```python
from build123d import *

# Parameters (mm, degrees)
MAINBLOCK_R                      = 2
MAINBLOCKBOSS_EXTRUDE1_DEPTH     = 23.4
TOPHOLECUT_SKETCH2_R             = 2.5
TOPHOLECUT_EXTRUDE1_DEPTH        = 45
MOUNTHOLEBORECUT_EXTRUDE2_DEPTH  = 2
TOPSPACERSKETCH4_R               = 3.5
TOPSPACERSKETCH4_R_2             = 2.5
TOPSPACERBOSS_EXTRUDE2_DEPTH     = 1
LOWERSPACERBOSS_EXTRUDE3_START   = 1
LOWERSPACERSKETCH5_R             = 3.5
LOWERSPACERSKETCH5_R_2           = 2.5
LOWERSPACERBOSS_EXTRUDE3_DEPTH   = 1
PUSHPINHOLESKETCH1_R             = 1
PUSHPINHOLECUT_EXTRUDE1_DEPTH    = 76.354665582
SCREWCOLLISIONSKETCH2_W          = 18.72
SCREWCOLLISIONSKETCH2_H          = 60
SCREWCOLLISIONCUT_EXTRUDE2_DEPTH = 5
SCREWCOLLISIONFILLET1_R          = 10
SCREWCOLLISIONFILLET2_R          = 10
MIDRAILINDENTSKETCH1_W           = 3.175
MIDRAILINDENTSKETCH1_H           = 40.4
MIDRAILINDENTCUT_EXTRUDE1_DEPTH  = 76.354665582


with BuildPart() as part:
    # MainBlock → MainBlockBoss-Extrude1 (new body)
    with BuildSketch(Plane.XY):
        Polygon((0, 0), (39.125, 0), (39.125, 19.8), (19.725, 19.8), (19.725, 40.2), (39.125, 40.2), (39.125, 60), (0, 60), align=None)
        with Locations((11.1125, 50.1)):
            Circle(MAINBLOCK_R, mode=Mode.SUBTRACT)
        with Locations((11.1125, 9.9)):
            Circle(MAINBLOCK_R, mode=Mode.SUBTRACT)
    extrude(amount=MAINBLOCKBOSS_EXTRUDE1_DEPTH)

    # TopHoleCut-Sketch2 → TopHoleCut-Extrude1 (cut)
    with BuildSketch(Plane(origin=(0, 60, 0), x_dir=(1, 0, 0), z_dir=(0, 1, 0))):
        with Locations(Location((29.425, -11.7, 0), (0, 0, 270))):
            Circle(TOPHOLECUT_SKETCH2_R)
    extrude(amount=-TOPHOLECUT_EXTRUDE1_DEPTH, mode=Mode.SUBTRACT)

    # MountHoleBoreSketch3 → MountHoleBoreCut-Extrude2 (cut)
    with BuildSketch(Plane.XY.offset(23.4)):
        Polygon((14.9875, 50.1), (13.05, 53.45584844), (9.175, 53.45584844), (7.2375, 50.1), (9.175, 46.74415156), (13.05, 46.74415156), align=None)
        Polygon((14.9875, 9.9), (13.05, 13.25584844), (9.175, 13.25584844), (7.2375, 9.9), (9.175, 6.54415156), (13.05, 6.54415156), align=None)
    extrude(amount=-MOUNTHOLEBORECUT_EXTRUDE2_DEPTH, mode=Mode.SUBTRACT)

    # TopSpacerSketch4 → TopSpacerBoss-Extrude2 (add)
    with BuildSketch(Plane.XZ.offset(-40.2)):
        with Locations(Location((29.425, 11.7, 0), (0, 0, 90))):
            Circle(TOPSPACERSKETCH4_R)
        with Locations(Location((29.425, 11.7, 0), (0, 0, 90))):
            Circle(TOPSPACERSKETCH4_R_2, mode=Mode.SUBTRACT)
    extrude(amount=TOPSPACERBOSS_EXTRUDE2_DEPTH)

    # LowerSpacerSketch5 → LowerSpacerBoss-Extrude3 (add)
    with BuildSketch(Plane(origin=(0, 19.8, 0), x_dir=(1, 0, 0), z_dir=(0, 1, 0)).offset(LOWERSPACERBOSS_EXTRUDE3_START)):
        with Locations(Location((29.425, -11.7, 0), (0, 0, 270))):
            Circle(LOWERSPACERSKETCH5_R)
        with Locations(Location((29.425, -11.7, 0), (0, 0, 270))):
            Circle(LOWERSPACERSKETCH5_R_2, mode=Mode.SUBTRACT)
    extrude(amount=-LOWERSPACERBOSS_EXTRUDE3_DEPTH)

    # PushPinHoleSketch1 → PushPinHoleCut-Extrude1 (cut, through all)
    with BuildSketch(Plane.XZ):
        with Locations(Location((29.425, 11.7, 0), (0, 0, 270))):
            Circle(PUSHPINHOLESKETCH1_R)
    extrude(amount=-PUSHPINHOLECUT_EXTRUDE1_DEPTH, mode=Mode.SUBTRACT)

    # ScrewCollisionSketch2 → ScrewCollisionCut-Extrude2 (cut)
    with BuildSketch(Plane.ZY):
        with Locations((9.36, 30)):
            Rectangle(SCREWCOLLISIONSKETCH2_W, SCREWCOLLISIONSKETCH2_H)
    extrude(amount=-SCREWCOLLISIONCUT_EXTRUDE2_DEPTH, mode=Mode.SUBTRACT)

    # ScrewCollisionFillet1
    # the kernel refuses this fillet: 10 mm, written as the material it adds along each edge
    with BuildSketch(Plane(origin=(5, 60, 18.72), x_dir=(-1, 0, 0), z_dir=(0, -1, 0))) as screwcollisionfillet1_piece_1:
        with BuildLine():
            CenterArc((10, 8.660254038), SCREWCOLLISIONFILLET1_R, 180, 60)
            Line((0, 8.660254038), (-0.2, 8.660254038))
            Line((-0.2, 8.660254038), (-0.2, 0))
            Line((-0.2, 0), (0, -0.2))
            ThreePointArc((0, -0.2), (2.5, -0.2), (4.9, -0.173205081))
            Line((4.9, -0.173205081), (5, 0))
        make_face()
    extrude(amount=60)

    # ScrewCollisionFillet2
    screwcollisionfillet2_edges = [part.edges().sort_by_distance(p)[0] for p in [
        (0, 30, 18.72),
    ]]
    fillet(screwcollisionfillet2_edges, radius=SCREWCOLLISIONFILLET2_R)

    # MidRailIndentSketch1 → MidRailIndentCut-Extrude1 (cut, through all)
    with BuildSketch(Plane.XY.offset(23.4)):
        with Locations((1.5875, 20.2)):
            Rectangle(MIDRAILINDENTSKETCH1_W, MIDRAILINDENTSKETCH1_H)
    extrude(amount=-MIDRAILINDENTCUT_EXTRUDE1_DEPTH, mode=Mode.SUBTRACT)


solid = part.part
```
The listing builds one solid part. Answer for the finished solid, in the listing's coordinates (mm). A direction names the side the tool comes from. Coordinates: 2 decimals unless noted, no trailing zeros. Write each loop counter-clockwise with the first axis right and the second up, starting at its lowest first coordinate (ties: lowest second). Pieces come first, ordered by that corner, then holes.
Q1. Section C-C, the plane y = 11 is taken. Write down the section's boundary in (x, z) (3 decimals), then the cut area to 3 significant figures.
Returned:
outline: (3.175, 15.819) arc R10 cw to (5, 10.06) - (5, 0) - (9.442, 0) - (9.442, 21.4) - (7.873, 21.4) - (7.873, 23.4) - (3.175, 23.4) - close; (12.783, 0) - (39.125, 0) - (39.125, 23.4) - (14.352, 23.4) - (14.352, 21.4) - (12.783, 21.4) - close; hole circle Ø2 at (29.425, 11.7)
area: 728 mm2
Q2. Section A-A, the plane z = 11.7 is taken. Give the number of separate pieces and of enclosed holes in the cut face, then the cut area to 3 significant figures.
Returned:
separate pieces: 3
enclosed holes: 2
area: 1,490 mm2
Q3. Section D-D, the plane z = 6 is taken. Write down the section's boundary in (x, y) (1 decimal).
Returned:
outline: (5, 0) - (39.1, 0) - (39.1, 19.8) - (19.7, 19.8) - (19.7, 40.2) - (39.1, 40.2) - (39.1, 60) - (5, 60) - close; hole circle Ø4 at (11.1, 9.9); hole circle Ø4 at (11.1, 50.1)
Q4. Section B-B, the plane x = 34 is taken. Write down the section's boundary in (y, z).
Returned:
outline: (0, 0) - (19.8, 0) - (19.8, 23.4) - (0, 23.4) - close; (40.2, 0) - (60, 0) - (60, 23.4) - (40.2, 23.4) - close
Q5. Find the intervals of material crossed by line 1 along Y through (x, z) = (11, 7.25); line 2 along Y through (x, z) = (30, 22.5); line 3 along Y through (x, z) = (13.5, 22), in increasing order.
Returned:
line 1: y = 0 to 7.9, 11.9 to 48.1, 52.1 to 60
line 2: y = 0 to 19.8, 40.2 to 60
line 3: y = 0 to 7.32, 12.48 to 47.52, 52.68 to 60
Q6. Given P1, Ø1, axis at x = 10.5, z = 22, coming from the -Y side; P2, Ø1.5, axis at x = 30, z = 10.5, coming from the +Y side; P3, Ø5, axis at y = 41.5, z = 6, coming from the -X side; P4, Ø8, axis at y = 25, z = 14, coming from the -X side (3 decimals), each flat-ended and moving along its own axis, determine where each tip first touches the part or whether it passes through.
Returned:
P1: stops at y = 0
P2: stops at y = 15
P3: stops at x = 5
P4: stops at x = 3.175
Q7. Which of the six approach directions +Z, -Z, +X, -X, +Y, -Y give full straight-line access (tool end or side, diameter ignored) to faces 4 (the cylindrical face through (26.984, 17.941, 11.158)), 5 (the flat face through (32, 19.8, 9)), 6 (the flat face through (29, 39.2, 9)), 7 (the flat face through (8.19, 48.45, 22.41))?
Returned:
face 4: +Y
face 5: none
face 6: +Z, -Z, +X
face 7: +Z
Q8. The mould has two halves that part along X. Classify faces 1 (the flat face through (39.125, 10, 12)), 2 (the cylindrical face through (26.32, 20.307, 13.315)), 3 (the flat face through (21, 0, 12)): released by +X, released by -X, zero draft, split by the parting line, or undercut.
Returned:
face 1: released by +X
face 2: undercut
face 3: zero draft
